Geometry check sheet. Reference: drawing and pictorial views, mm from the part's lowest x, y, z. Round coordinates to 2 decimals unless told otherwise and drop trailing zeros. Loops run counter-clockwise (first coordinate to the right, second up) from the corner with the lowest first, then second, coordinate; pieces in that order, holes last. Notation, with made-up numbers: (-18.5, 53) -> (37.5, 53) arc R20 cw to (37.5, 85) -> close; hole circle Ø4 at (-10.5, 36). An arc over 180 degrees is marked (long way). Use one line per item in the form item = value. Start each with the question number.
(1) Sectioned sample at C-C (x = 39.5). Record the cut outline in (y, z), and give its area (3 significant figures).
(2) Sectioned sample at D-D (y = 5). Record the cut outline in (x, z).
(3) Go/stop test with flat-tipped pins: pin 1 (4.5 mm diameter, centred on x = 11.176, z = 11.176, fed in from +Y); pin 2 (5 mm diameter, centred on y = 3, z = 34, fed in from +X); pin 3 (8 mm diameter, centred on y = 5, z = 20.5, fed in from -X); pin 4 (1.5 mm diameter, centred on x = 19.5, y = 8.5, fed in from -Z). Record where each tip stops, or that it passes through.
(4) Draft check along X on the marked faces 1, 2 and 3. Enter one of: released by +X, released by -X, zero draft, split by the parting line, or undercut.
(5) Sectioned sample at A-A (x = 32.5). Record the cut outline in (y, z), and give its area (3 significant figures).
(6) Material ranges on probe 1 along X at (y, z) = (13, 39); probe 2 along Z at (x, y) = (10, 3.25); probe 3 along Z at (x, y) = (40, 9.5), recorded low to high. Write a range as [from, to].
(7) Sectioned sample at B-B (z = 14). Record the cut outline in (x, y).
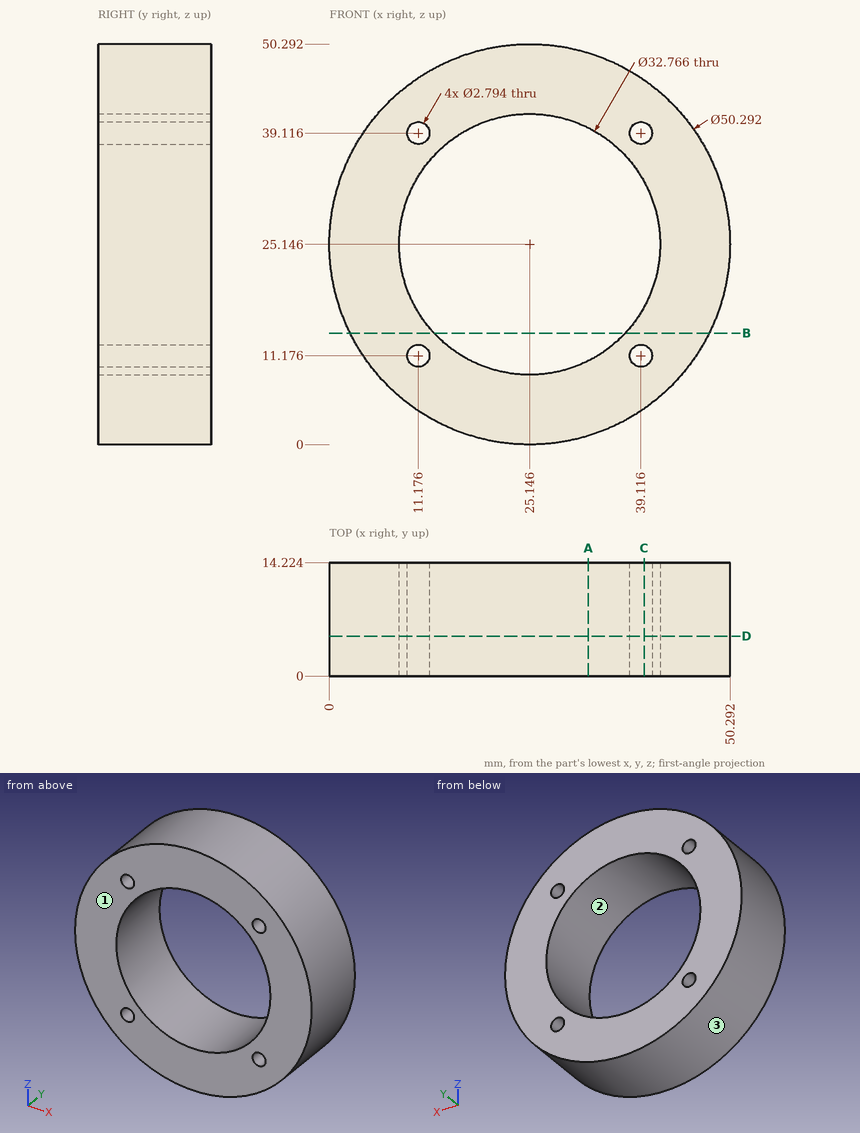
Checks:
q1.outline = (0, 4.5) -> (14.22, 4.5) -> (14.22, 9.83) -> (0, 9.83) -> close; (0, 12.52) -> (14.22, 12.52) -> (14.22, 17.25) -> (0, 17.25) -> close; (0, 33.04) -> (14.22, 33.04) -> (14.22, 37.77) -> (0, 37.77) -> close; (0, 40.46) -> (14.22, 40.46) -> (14.22, 45.79) -> (0, 45.79) -> close
q1.area = 286 mm2
q2.outline = circle Ø50.29 at (25.15, 25.15); hole circle Ø32.77 at (25.15, 25.15); hole circle Ø2.79 at (11.18, 11.18); hole circle Ø2.79 at (11.18, 39.12); hole circle Ø2.79 at (39.12, 11.18); hole circle Ø2.79 at (39.12, 39.12)
q3.pin_1 = 14.22
q3.pin_2 = 49.48
q3.pin_3 = 0.01
q3.pin_4 = 0.48
q4.face_1 = zero draft
q4.face_2 = undercut
q4.face_3 = split by the parting line
q5.outline = (0, 1.1) -> (14.22, 1.1) -> (14.22, 10.51) -> (0, 10.51) -> close; (0, 39.79) -> (14.22, 39.79) -> (14.22, 49.19) -> (0, 49.19) -> close
q5.area = 268 mm2
q6.probe_1 = [4.16, 9.78], [12.57, 16.4], [33.89, 37.72], [40.51, 46.13]
q6.probe_2 = [5.07, 10.42], [11.93, 18.9], [31.39, 38.36], [39.87, 45.22]
q6.probe_3 = [4.86, 10.09], [12.26, 18.24], [32.06, 38.03], [40.2, 45.44]
q7.outline = (2.61, 0) -> (13.14, 0) -> (13.14, 14.22) -> (2.61, 14.22) -> close; (37.15, 0) -> (47.69, 0) -> (47.69, 14.22) -> (37.15, 14.22) -> close
